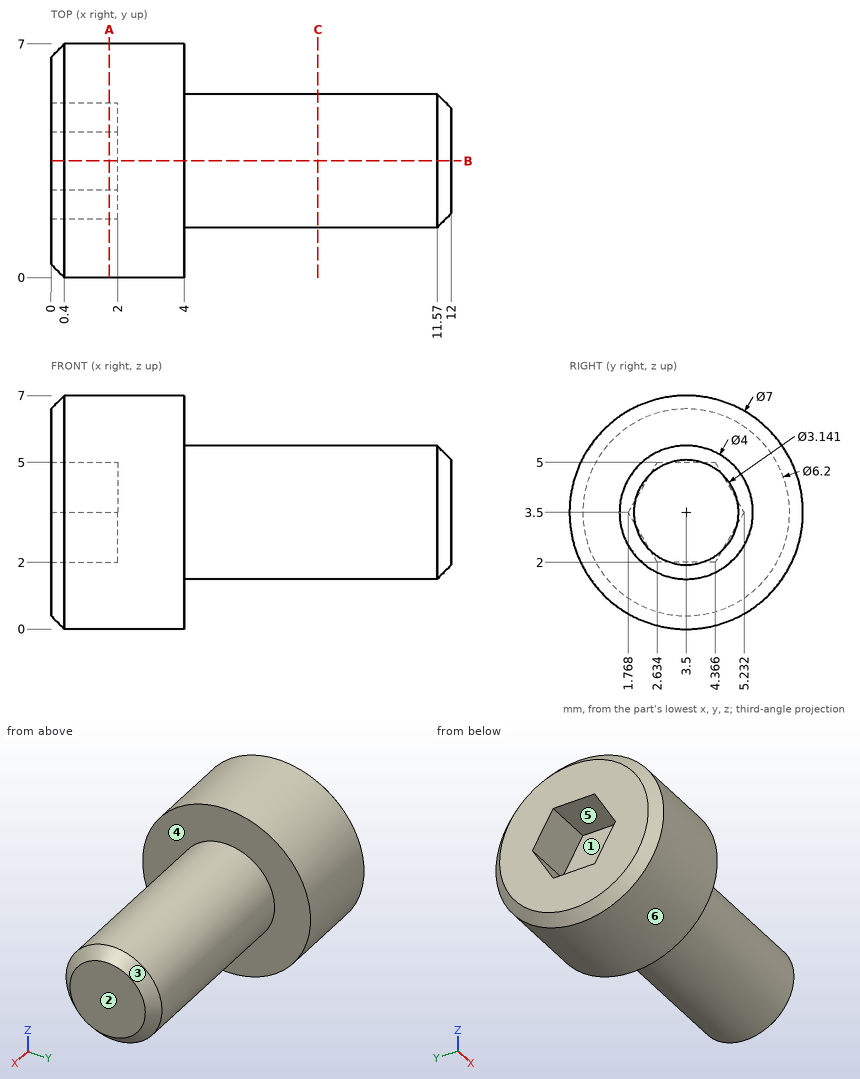
Can you work these out from the drawing? Everything is in mm from the part's minimum corner. A direction names the side the tool comes from. Round coordinates to 2 decimals unless told otherwise and drop trailing zeros. Loops run counter-clockwise (first coordinate to the right, second up) from the corner with the lowest first, then second, coordinate; pieces in that order, holes last. Notation, with made-up numbers: (-1, 39) -> (50, 39) arc R24 ccw to (50, 78) -> close; hole circle Ø8 at (-5.5, -8). An arc over 180 degrees is marked (long way). Use CSV: the item, a comma, the result in double quotes.
(1) Suppose I cut it at B-B on y = 3.5. Write out the boundary of the cut face in (x, z).
Return value:
outline,"(0, 0.4) -> (0.4, 0) -> (4, 0) -> (4, 1.5) -> (11.57, 1.5) -> (12, 1.93) -> (12, 5.07) -> (11.57, 5.5) -> (4, 5.5) -> (4, 7) -> (0.4, 7) -> (0, 6.6) -> (0, 5) -> (2, 5) -> (2, 2) -> (0, 2) -> close"
(2) Will these pins go through, and if not, where does the flat tip stop? pin 1 Ø4 at (x, y) = (8.5, 4) entering from -Z; pin 2 Ø0.5 at (x, y) = (1.5, 4) entering from +Z; pin 3 Ø2 at (x, z) = (6.5, 3) entering from -Y.
Return value:
pin 1,"stops at z = 1.5"
pin 2,"stops at z = 6.99"
pin 3,"stops at y = 1.5"
(3) If we mould it in two halves opening along Z, with no side actions, what happens to the marked faces 1, 2 and 3? For each: +Z half, -Z half, draft (parallel to the pull), parting line (faces both ways), or undercut.
Return value:
face 1,"undercut"
face 2,"draft"
face 3,"parting line"
(4) For the marked faces 4, 5 and 6, which set-ups out of +Z, -Z, +X, -X, +Y, -Y let a thin tool reach every point of the face, with its end or its side?
Return value:
face 4,"+X"
face 5,"-X"
face 6,"+X, -X"
(5) Suppose I cut it at A-A on x = 1.75. Write out the boundary of the cut face in (y, z).
Return value:
outline,"circle Ø7 at (3.5, 3.5); hole (1.77, 3.5) -> (2.63, 2) -> (4.37, 2) -> (5.23, 3.5) -> (4.37, 5) -> (2.63, 5) -> close"
(6) If I drill on probe 1 along X at (y, z) = (2.75, 5.5); probe 2 along Z at (x, y) = (7.5, 4.5); probe 3 along X at (y, z) = (2.5, 3.25), over which ranges is the centre line in solid material (lowest first)? Write a range as [from, to].
Return value:
probe 1,"x = [0, 4]"
probe 2,"z = [1.77, 5.23]"
probe 3,"x = [2, 12]"
(7) Suppose I cut it at C-C on x = 8. Write out the boundary of the cut face in (y, z).
Return value:
outline,"circle Ø4 at (3.5, 3.5)"
